For this review, take the finished solid that the model builds, in its own axes (mm). A direction names the side the tool comes from. Give positions to 0.01 mm unless a question says otherwise; leave off trailing zeros. Write each loop counter-clockwise with the first axis right and the second up, starting at its lowest first coordinate (ties: lowest second). Pieces come first, ordered by that corner, then holes.
1) We need section B-B on z = 15. Give the boundary of the cut face in (x, y), and give its area (3 significant figures).
2) For P1, Ø3.5, axis at x = 2.5, y = -15, coming from the +Z side; P2, Ø2, axis at y = -14.5, z = 5.5, coming from the -X side; P3, Ø3, axis at x = 27, z = 3, coming from the +Y side; P4, Ø1.1, axis at x = 2.5, z = 4.5, coming from the +Y side, all flat-tipped, find the tip position at first contact; note any pin that passes through.
3) We need section D-D on y = -8.5. Give the boundary of the cut face in (x, z), and give its area (3 significant figures).
4) Draft analysis for pull direction X (two halves, no side actions). For faces 6 (the face through (-27.092, 0.601, 2.535)), 7 (the face through (-25, 8, 2)), 8 (the face through (27, 4, 3)), state which applies: pulls with the +X half, pulls with the -X half, needs draft (parallel to the pull), parting line crosses it, or undercut.
5) We need section A-A on x = 0. Give the boundary of the cut face in (y, z), and give its area (3 significant figures).
6) Wall thickness on line 1 along Z through (x, y) = (-2, -9); line 2 along Y through (x, z) = (29, 1.5); line 3 along Z through (x, y) = (0, -43.25): over which ranges is each line inside the solid? List them lowest first.
7) Machinability: for faces 1 (the face through (0, -15, 4)), 2 (the face through (0, 10, 4)), 3 (the face through (-21, -12.5, 2)), 4 (the face through (27, -4, 3)), 5 (the face through (25, 8, 2)), which of the approach directions +Z, -Z, +X, -X, +Y, -Y give a long, thin tool a straight path to every point of the face, cutting with its end or side? Answer none if there is none.
8) We need section C-C on z = 2. Give the boundary of the cut face in (x, y), and give its area (3 significant figures).
from build123d import *

# Parameters (mm, degrees)
SKETCH_W         = 50
SKETCH_H         = 25
PAD_DEPTH        = 5
PAD001_DEPTH     = 5
SKETCH002_R      = 2
POCKET_DEPTH     = 131.713272
SKETCH004_W      = 12
SKETCH004_H      = 5
POCKET001_DEPTH  = 1
PAD002_DEPTH     = 5
SKETCH008_W      = 8
SKETCH008_H      = 10
POCKET002_DEPTH  = 1
SKETCH009_W      = 12
SKETCH009_H      = 10
POCKET003_DEPTH  = 1
PAD003_DEPTH     = 20
HOLE_D           = 3.4
HOLE_DEPTH       = 25
HOLE_CSINK_D     = 6.1
HOLE_CSINK_ANGLE = 90
HOLE_TIPS_R      = 1.7


with BuildPart() as part:
    # Sketch → Pad (new body)
    with BuildSketch(Plane.XY):
        Rectangle(SKETCH_W, SKETCH_H)
    extrude(amount=PAD_DEPTH)

    # Sketch001 (on Face6 of Pad) → Pad001 (join)
    with BuildSketch(Plane.XY.offset(5)):
        with BuildLine():
            ThreePointArc((-25, -4), (-21, 0), (-25, 4))
            Line((-25, 4), (-29, 4))
            ThreePointArc((-29, 4), (-33, 0), (-29, -4))
            Line((-25, -4), (-29, -4))
        make_face()
    pad001 = extrude(amount=-PAD001_DEPTH)

    # Sketch002 (on Face12 of Pad001) → Pocket (cut, through all)
    with BuildSketch(Plane.XY.offset(5)):
        with Locations((-29, 0)):
            Circle(SKETCH002_R)
    pocket = extrude(amount=-POCKET_DEPTH, mode=Mode.SUBTRACT)

    # Mirrored: Pad001 across Sketch001 V_Axis
    add(pad001.mirror(Plane(origin=(0, 0, 5), x_dir=(0, 0, 1), z_dir=(1, 0, 0))))

    # Mirrored001: Pocket across Sketch002 V_Axis
    add(pocket.mirror(Plane(origin=(0, 0, 5), x_dir=(0, 0, 1), z_dir=(1, 0, 0))), mode=Mode.SUBTRACT)

    # Sketch004 (on Face5 of Mirrored001) → Pocket001 (cut)
    with BuildSketch(Plane.XY.offset(5)):
        with Locations((0, 10)):
            Rectangle(SKETCH004_W, SKETCH004_H)
    pocket001 = extrude(amount=-POCKET001_DEPTH, mode=Mode.SUBTRACT)

    # Mirrored002: Pocket001 across Sketch004 H_Axis
    add(pocket001.mirror(Plane(origin=(0, 0, 5), x_dir=(0, 0, 1), z_dir=(0, 1, 0))), mode=Mode.SUBTRACT)

    # Sketch005 (on Face2 of Mirrored002) → Pad002 (join)
    with BuildSketch(Plane(origin=(0, 0, 0), x_dir=(1, 0, 0), z_dir=(0, 0, -1))):
        Polygon((-17, 12.5), (-7, 49.820508), (7, 49.820508), (17, 12.5), align=None)
    extrude(amount=-PAD002_DEPTH)

    # Sketch008 → Pocket002 (cut)
    with BuildSketch(Plane(origin=(-25, 0, 0), x_dir=(0, -1, 0), z_dir=(-1, 0, 0))):
        with Locations((0, -5)):
            Rectangle(SKETCH008_W, SKETCH008_H)
    extrude(amount=-POCKET002_DEPTH, mode=Mode.SUBTRACT)

    # Sketch009 (on Face17 of Pad002) → Pocket003 (cut)
    with BuildSketch(Plane.XY.offset(5)):
        with Locations((0, -17.5)):
            Rectangle(SKETCH009_W, SKETCH009_H)
    extrude(amount=-POCKET003_DEPTH, mode=Mode.SUBTRACT)

    # Sketch010 (on Face19 of Pocket003) → Pad003 (join)
    with BuildSketch(Plane.XY.offset(5)):
        Polygon((-7, -49.820508), (7, -49.820508), (9.679492, -39.820508), (-9.679492, -39.820508), align=None)
    extrude(amount=PAD003_DEPTH)

    # Hole
    with Locations(Plane.XZ.offset(49.820508)):
        with Locations((0, 15)):
            CounterSinkHole(HOLE_D / 2, HOLE_CSINK_D / 2, depth=HOLE_DEPTH, counter_sink_angle=HOLE_CSINK_ANGLE)

    # Hole tips → Hole tip 1 section 0
    with BuildSketch(Plane.XZ.offset(24.820508), mode=Mode.PRIVATE) as hole_tip_1_s0:
        with Locations((0, 15)):
            Circle(HOLE_TIPS_R)
    loft([hole_tip_1_s0.sketch, Vertex(0, -23.799045, 15)], mode=Mode.SUBTRACT)


solid = part.part
Results list:
1. outline: (-9.68, -39.82) - (-7, -49.82) - (-3.05, -49.82) - (-1.7, -48.47) - (-1.7, -39.82) - close; (1.7, -48.47) - (3.05, -49.82) - (7, -49.82) - (9.68, -39.82) - (1.7, -39.82) - close
1. area: 131 mm2
2. P1: stops at z = 4
2. P2: stops at x = -16.7
2. P3: stops at y = 4
2. P4: stops at y = 12.5
3. outline: (-25, 0) - (25, 0) - (25, 5) - (6, 5) - (6, 4) - (-6, 4) - (-6, 5) - (-25, 5) - close
3. area: 238 mm2
4. face 6: undercut
4. face 7: pulls with the -X half
4. face 8: needs draft
5. outline: (-49.82, 0) - (12.5, 0) - (12.5, 4) - (7.5, 4) - (7.5, 5) - (-7.5, 5) - (-7.5, 4) - (-22.5, 4) - (-22.5, 5) - (-39.82, 5) - (-39.82, 13.3) - (-48.47, 13.3) - (-49.82, 11.95) - close; (-49.82, 18.05) - (-48.47, 16.7) - (-39.82, 16.7) - (-39.82, 25) - (-49.82, 25) - close
5. area: 456 mm2
6. line 1: z = 0 to 4
6. line 2: y = -4 to -2, 2 to 4
6. line 3: z = 0 to 13.3, 16.7 to 25
7. face 1: +Z
7. face 2: +Z, +Y
7. face 3: +Z, -Z, -X, -Y
7. face 4: +Z, -Z, +X, -Y
7. face 5: +Z, -Z, +X, +Y
8. outline: (-29, -4) - (-25, -4) - (-25, -12.5) - (-17, -12.5) - (-7, -49.82) - (7, -49.82) - (17, -12.5) - (25, -12.5) - (25, -4) - (29, -4) arc R4 ccw to (29, 4) - (25, 4) - (25, 12.5) - (-25, 12.5) - (-25, 4) - (-29, 4) arc R4 ccw to start; hole circle Ø4 at (-29, 0); hole circle Ø4 at (29, 0)
8. area: 2,230 mm2
